```python
from build123d import *

# Parameters (mm, degrees)
CHAMFER_1_SIZE      = 2
SKETCH_2_R          = 5
CUT_EXTRUDE_1_DEPTH = 162.952153428
CHAMFER_2_SIZE      = 0.25


with BuildPart() as part:
    # 草图1 → 旋转1 (revolve)
    with BuildSketch(Plane.XY, mode=Mode.PRIVATE) as revolve_1_sk:
        Polygon((0, 0), (0, 36.5), (8, 36.5), (8, 30.25), (128, 30.25), (138, 24.5), (138, 0), align=None)
    revolve(revolve_1_sk.sketch.rotate(Axis((0, 0, 0), (1, 0, 0)), 90), axis=Axis((0, 0, 0), (1, 0, 0)))

    # 倒角1
    chamfer_1_edges = [part.edges().sort_by_distance(p)[0] for p in [
        (0, 0, -36.5),
    ]]
    chamfer(chamfer_1_edges, length=CHAMFER_1_SIZE)

    # 草图2 → 切除-拉伸1 (cut, through all)
    with BuildSketch(Plane.XY.offset(40)):
        with Locations((118, 0)):
            Circle(SKETCH_2_R)
    extrude(amount=-CUT_EXTRUDE_1_DEPTH, mode=Mode.SUBTRACT)

    # 倒角2
    chamfer_2_edges = [part.edges().sort_by_distance(p)[0] for p in [
        (8, 0, -36.5),
    ]]
    chamfer(chamfer_2_edges, length=CHAMFER_2_SIZE)


solid = part.part
```
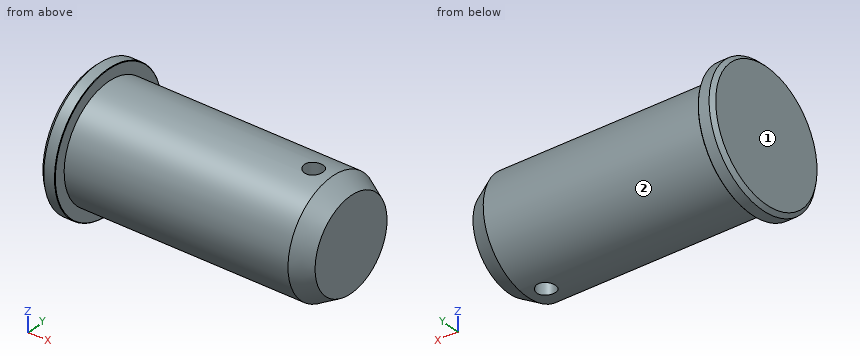
Part model, mm, in its own coordinate system. Face numbers are marked on the shaded views. A direction names the side the tool comes from. Coordinates: 2 decimals unless noted, no trailing zeros. Order: outer loops, then holes, each group sorted by start corner. A loop starts at its lowest first (then second) coordinate and runs counter-clockwise, first axis right, second up. Notation, with made-up numbers: (80, 30.25) -> (98, 30.25) arc R20 ccw to (98, 67.25) -> close; hole circle Ø1 at (50.5, 32.5). An arc over 180 degrees is marked (long way). Put each result on its own line as item: value. Start each with the question number.
(1) Pin check, flat tips, straight feed: pin 1 Ø10 at (x, z) = (77, 13) entering from -Y; pin 2 Ø1.5 at (x, y) = (15.5, 26) entering from +Z; pin 3 Ø12 at (x, z) = (102, -25.5) entering from -Y. Stop position of each tip, or through.
(2) Band-saw the part on D-D (x = 118). Give the cut face in (y, z), then the cut area to 3 significant figures.
(3) Probe line 1 along X through (y, z) = (0, 12); line 2 along Z through (x, y) = (62.5, 1); line 3 along X through (y, z) = (-3, 32.5). List the from-to ranges inside material, lowest first. Write a range as [from, to].
(4) Band-saw the part on C-C (x = 47). Give the cut face in (y, z), then the cut area to 3 significant figures.
(5) Band-saw the part on A-A (y = 0). Give the cut face in (x, z), then the cut area to 3 significant figures.
(6) Band-saw the part on B-B (z = 0). Give the cut face in (x, y).
(7) Which spindle directions (+Z, -Z, +X, -X, +Y, -Y) get a long thin tool onto all of the face, cutting with end or side? Do the marked faces 1 and 2. Say none if no direction does.
Determined:
1. pin 1: stops at y = -29.17
1. pin 2: stops at z = 16.66
1. pin 3: stops at y = -23.13
2. outline: (-5, -29.83) -> (-5, 29.83) arc R30.25 ccw to start; (5, -29.83) arc R30.25 ccw to (5, 29.83) -> close
2. area: 2,270 mm²
3. line 1: x = [0, 113], [123, 138]
3. line 2: z = [-30.23, 30.23]
3. line 3: x = [0, 8]
4. outline: circle Ø60.5 at (0, 0)
4. area: 2,870 mm²
5. outline: (0, -34.5) -> (2, -36.5) -> (7.75, -36.5) -> (8, -36.25) -> (8, -30.25) -> (113, -30.25) -> (113, 30.25) -> (8, 30.25) -> (8, 36.25) -> (7.75, 36.5) -> (2, 36.5) -> (0, 34.5) -> close; (123, -30.25) -> (128, -30.25) -> (138, -24.5) -> (138, 24.5) -> (128, 30.25) -> (123, 30.25) -> close
5. area: 7,780 mm²
6. outline: (0, -34.5) -> (2, -36.5) -> (7.75, -36.5) -> (8, -36.25) -> (8, -30.25) -> (128, -30.25) -> (138, -24.5) -> (138, 24.5) -> (128, 30.25) -> (8, 30.25) -> (8, 36.25) -> (7.75, 36.5) -> (2, 36.5) -> (0, 34.5) -> close; hole circle Ø10 at (118, 0)
7. face 1: +Z, -Z, -X, +Y, -Y
7. face 2: +X
